Part print with two shaded views. Sizes in mm from the minimum x, y, z corner. A direction names the side the tool comes from. Round coordinates to 2 decimals unless told otherwise and drop trailing zeros. Loops run counter-clockwise (first coordinate to the right, second up) from the corner with the lowest first, then second, coordinate; pieces in that order, holes last. Notation, with made-up numbers: (34, 23) - (74, 23) arc R17 ccw to (74, 34) - close; hole circle Ø7 at (28, 9). An arc over 180 degrees is marked (long way). Write each question's results on one line, items separated by ' | '. Start each with the question number.
(1) Cut at C-C, the plane z = 10. List the corners of the cut face in (x, y) (1 decimal).
(2) Mould opens along Y. For the marked faces 3 and 4 say: released by +Y, released by -Y, zero draft, split by the parting line, or undercut.
(3) Tool access for the marked faces 1 and 2: list every direction of +Z, -Z, +X, -X, +Y, -Y with a clear straight run to the whole face (end or side of a thin tool).
(4) Flat gauge pins, fed straight in: P1, Ø0.6, axis at x = 14, y = 43.5, coming from the +Z side; P2, Ø1.5, axis at y = 6.5, z = 3.5, coming from the +X side; P3, Ø12, axis at x = 10, y = 27, coming from the +Z side; P4, Ø1, axis at y = 15.5, z = 2, coming from the +X side. Where does each tip first touch, or does it go through?
(5) Cut at B-B, the plane x = 22. List the corners of the cut face in (y, z).
(6) Cut at D-D, the plane y = 18.5. List the corners of the cut face in (x, z), then the cut area to 3 significant figures.
(7) Drill centre lines: L1, parallel to Y at x = 6.25, z = 6.25 (1 decimal); L2, parallel to Z at x = 10.5, y = 33.5; L3, parallel to X at y = 36.5, z = 4 (1 decimal). Where is each one in solid material? Low to high.
(8) Cut at A-A, the plane z = 2.75. Give the number of separate pieces and of enclosed holes in the cut face.
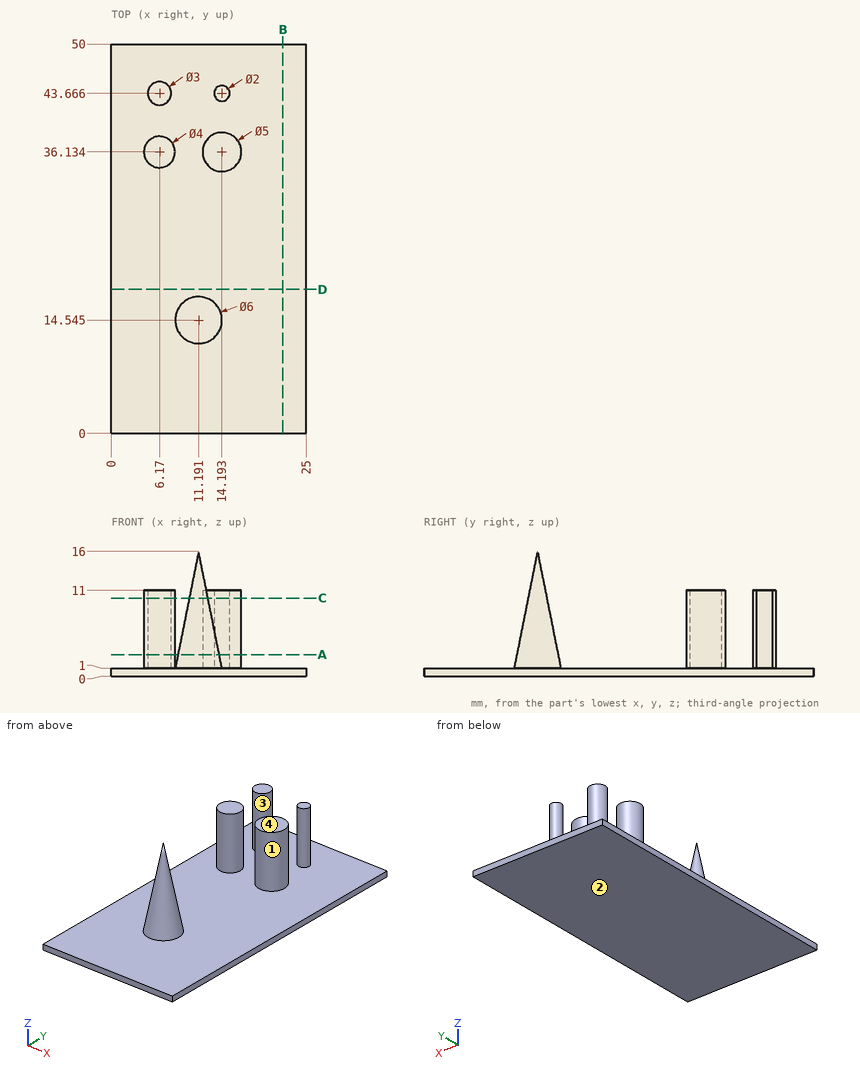
A:
1) outline: circle Ø4 at (6.2, 36.1); circle Ø3 at (6.2, 43.7); circle Ø2.4 at (11.2, 14.5); circle Ø5 at (14.2, 36.1); circle Ø2 at (14.2, 43.7)
2) face 3: undercut | face 4: zero draft
3) face 1: +Z | face 2: -Z, +X, -X, +Y, -Y
4) P1: z = 11 | P2: through | P3: z = 1 | P4: x = 14
5) outline: (0, 0) - (50, 0) - (50, 1) - (0, 1) - close
6) outline: (0, 0) - (25, 0) - (25, 1) - (0, 1) - close | area: 25.0 mm2
7) L1: 34.1 to 38.1, 42.2 to 45.2 | L2: 0 to 1 | L3: 4.2 to 8.1, 11.7 to 16.7
8) separate pieces: 5 | enclosed holes: 0
